Work out the finished part from the listing and answer in its coordinate system (mm). Face numbers are marked on the shaded views. A direction names the side the tool comes from. Coordinates: 2 decimals unless noted, no trailing zeros. Loops run counter-clockwise (first coordinate to the right, second up) from the corner with the lowest first, then second, coordinate; pieces in that order, holes last. Notation, with made-up numbers: (37, 72) -> (54, 72) arc R20 ccw to (54, 90) -> close; hole circle Ø9 at (-16.5, -24.75). An arc over 180 degrees is marked (long way). One line per question, with ' | ' between items.
Autodesk Inventor part; units mm, degrees
ref_plane "YZ Plane" through (0, 0, 0) normal (1, 0, 0) x (0, 1, 0)
ref_plane "XZ Plane" through (0, 0, 0) normal (0, 1, 0) x (-1, 0, 0)
ref_plane "XY Plane" through (0, 0, 0) normal (0, 0, 1) x (1, 0, 0)
sketch "草图1" plane through (0, 0, 0) normal (0, 0, 1) x (1, 0, 0)
  line L0 (-195, 125) -> (195, 125)
  line L1 (195, 125) -> (195, -125)
  line L2 (195, -125) -> (-195, -125)
  line L3 (-195, -125) -> (-195, 125)
  line L4 (0, -175) -> (0, 175)
  line L5 (-273, 0) -> (273, 0)
  point P0 (0, 0)
  dimension "d0" = 250
  dimension "d1" = 390
extrude "拉伸1" add sketch "草图1" along normal mid plane 300
sketch "草图2" plane through (-195, 125, 150) normal (0, 1, 0) x (1, 0, 0)
  line L0 (15, 25) -> (375, 25)
  line L1 (375, 25) -> (375, 275)
  line L2 (375, 275) -> (15, 275)
  line L3 (15, 275) -> (15, 25)
  line L4 (-78, 150) -> (468, 150)
  line L5 (195, 360) -> (195, -60)
  point P0 (195, 150)
  dimension "d4" = 360
  dimension "d5" = 250
extrude "拉伸2" cut sketch "草图2" against normal blind 245
sketch "草图3" plane through (0, 0, 150) normal (0, 0, 1) x (1, 0, 0)
  line L0 (-50, 25) -> (50, 25)
  line L1 (50, 25) -> (50, -25)
  line L2 (50, -25) -> (-50, -25)
  line L3 (-50, -25) -> (-50, 25)
  line L4 (-273, 0) -> (273, 0)
  line L5 (0, -175) -> (0, 175)
  point P0 (0, 0)
  dimension "d8" = 100
  dimension "d9" = 50
extrude "拉伸3" cut sketch "草图3" against normal blind 17
sketch "草图4" plane through (0, 0, 150) normal (0, 0, 1) x (1, 0, 0)
  line L0 (-50, -25) -> (-50, 25)
  line L1 (50, 25) -> (50, -25)
  line L2 (-50, 25) -> (50, 25)
  line L3 (50, 25) -> (50, 0)
  line L4 (50, 0) -> (-50, 0)
  line L5 (-50, 0) -> (-50, 25)
  point P0 (0, 0)
extrude "拉伸4" add sketch "草图4" against normal blind 5
mirror "镜像1" about plane through (0, 0, 0) normal (0, 0, 1) of "拉伸3", "拉伸4"
chamfer "倒角1" distance 17 angle 45 2 edges at (0, -25, 150) (0, -25, -150)
chamfer "倒角2" distance 5 angle 45 2 edges at (0, 0, 145) (0, 0, -145)
properties part number "容器"
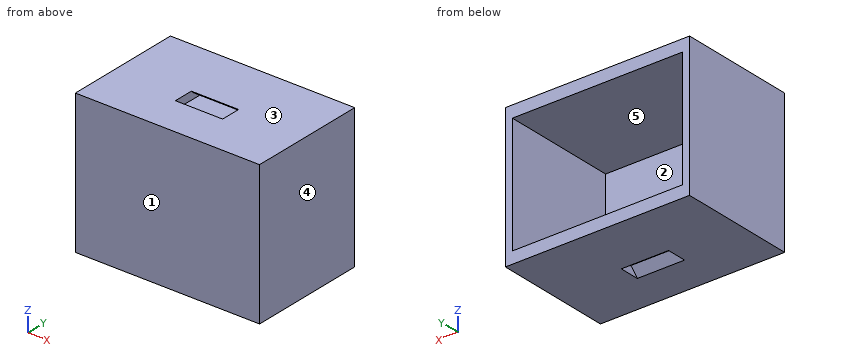
1) Find section C-C (z = 26). Write down the section's boundary in (x, y), plus the area to 3 significant figures.
Check values:
outline: (-195, -125) -> (195, -125) -> (195, 125) -> (180, 125) -> (180, -120) -> (-180, -120) -> (-180, 125) -> (-195, 125) -> close | area: 9,300 mm^2
2) A flat-ended cylindrical pin translates along its axis: pin 1 (1 mm diameter, centred on x = 44.5, z = 75.5, fed in from +Y). Find the tip coordinate at first contact, or state that the pin passes through.
Check values:
pin 1: stops at y = -120
3) Find section A-A (y = 13). Write down the section's boundary in (x, z).
Check values:
outline: (-195, -150) -> (195, -150) -> (195, 150) -> (-195, 150) -> close; hole (-180, -125) -> (180, -125) -> (180, 125) -> (-180, 125) -> close; hole (-50, -145) -> (50, -145) -> (50, -133) -> (-50, -133) -> close; hole (-50, 133) -> (50, 133) -> (50, 145) -> (-50, 145) -> close
4) The mould has two halves that part along Z. Classify the marked faces 1, 2 and 3: released by +Z, released by -Z, zero draft, split by the parting line, or undercut.
Check values:
face 1: zero draft | face 2: undercut | face 3: released by +Z
5) Find section D-D (y = -17). Write down the section's boundary in (x, z), plus the area to 3 significant figures.
Check values:
outline: (-195, -150) -> (-50, -150) -> (-50, -133) -> (50, -133) -> (50, -150) -> (195, -150) -> (195, 150) -> (50, 150) -> (50, 133) -> (-50, 133) -> (-50, 150) -> (-195, 150) -> close; hole (-180, -125) -> (180, -125) -> (180, 125) -> (-180, 125) -> close | area: 23,600 mm^2
6) For the marked faces 4 and 5, determine the directions among +Z, -Z, +X, -X, +Y, -Y from which every point of the face is accessible in a straight line to the end or side of a thin tool.
Check values:
face 4: +Z, -Z, +X, +Y, -Y | face 5: +Y
7) Find the intervals of material crossed by line 1 along Z through (x, y) = (51.5, 28.5); line 2 along Z through (x, y) = (31, -37); line 3 along X through (y, z) = (86, 69.5), in increasing order.
Check values:
line 1: z = -150 to -125, 125 to 150 | line 2: z = -145 to -125, 125 to 145 | line 3: x = -195 to -180, 180 to 195
